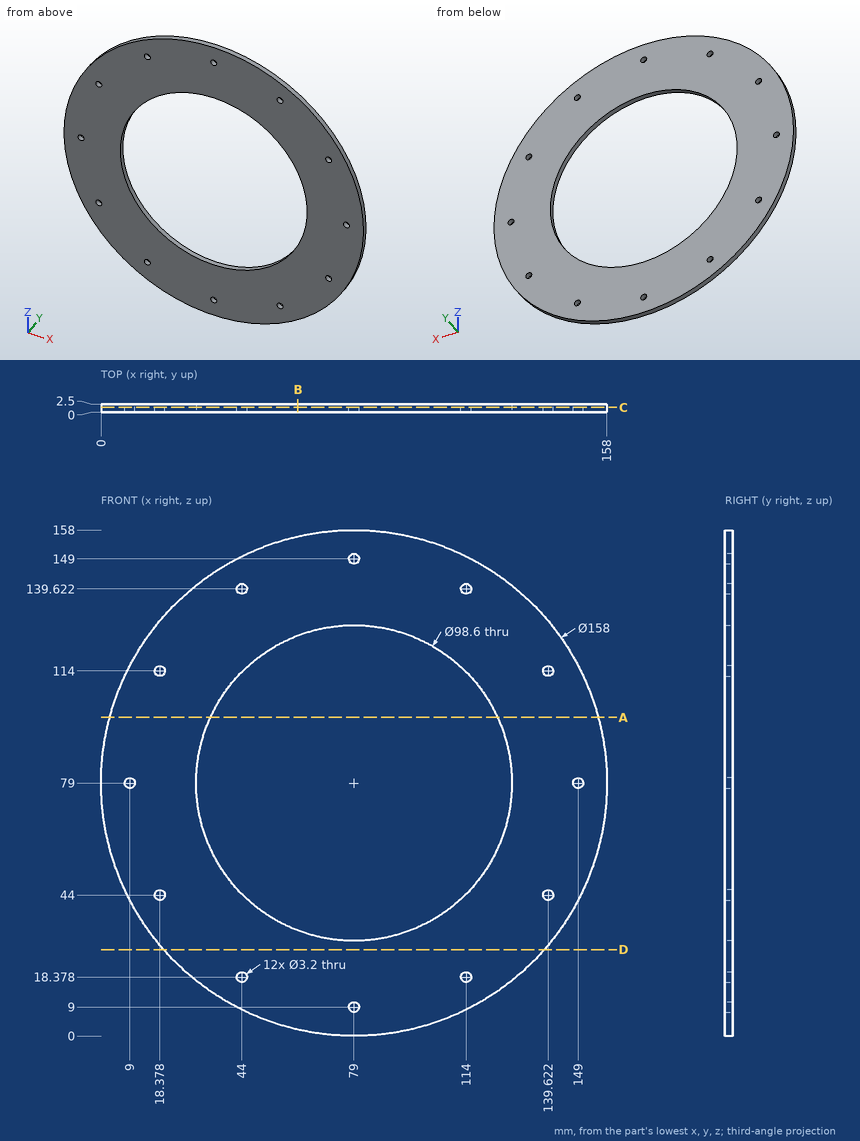
For this review, use the dimensioned drawing (mm, ordinates from the lowest corner) and the shaded views. Give positions to 0.01 mm unless a question says otherwise; leave off trailing zeros. Order: outer loops, then holes, each group sorted by start corner. A loop starts at its lowest first (then second) coordinate and runs counter-clockwise, first axis right, second up.
1) Take a section at D-D (z = 27). Give the boundary of the cut face in (x, y).
2) Insertion check: pin 1 (3.5 mm diameter, centred on x = 139.62, z = 114, fed in from -Y); pin 2 (1.9 mm diameter, centred on x = 149, z = 79, fed in from +Y); pin 3 (1 mm diameter, centred on x = 124, y = 1.5, fed in from -Z) (1 decimal); pin 4 (1.5 mm diameter, centred on y = 2, z = 52.5, fed in from -X). Each pin has a flat end and moves straight along its axis. Give the tip position at first contact, or say it passes through.
3) Wall thickness on line 1 (X direction, y = 0.5, z = 9); line 2 (X direction, y = 0.6, z = 18) (1 decimal); line 3 (X direction, y = 1.8, z = 80): over which ranges is each line inside the solid? List them lowest first.
4) Take a section at A-A (z = 99.5). Give the boundary of the cut face in (x, y), then the cut area to 3 significant figures.
5) Take a section at B-B (x = 61.5). Give the boundary of the cut face in (y, z), then the cut area to 3 significant figures.
6) Take a section at C-C (y = 1.45). State how many separate pieces and enclosed holes the cut face has, then the cut area to 3 significant figures.
Derived:
1. outline: (19.53, 0) - (138.47, 0) - (138.47, 2.5) - (19.53, 2.5) - close
2. pin 1: stops at y = 0
2. pin 2: passes through
2. pin 3: stops at z = 13.7
2. pin 4: stops at x = 4.31
3. line 1: x = 42.38 to 77.4, 80.6 to 115.62
3. line 2: x = 28.8 to 42.4, 45.6 to 112.4, 115.6 to 129.2
3. line 3: x = 0.01 to 7.75, 10.25 to 29.71, 128.29 to 147.75, 150.25 to 157.99
4. outline: (2.71, 0) - (34.16, 0) - (34.16, 2.5) - (2.71, 2.5) - close; (123.84, 0) - (155.29, 0) - (155.29, 2.5) - (123.84, 2.5) - close
4. area: 157 mm2
5. outline: (0, 1.96) - (2.5, 1.96) - (2.5, 32.91) - (0, 32.91) - close; (0, 125.09) - (2.5, 125.09) - (2.5, 156.04) - (0, 156.04) - close
5. area: 155 mm2
6. separate pieces: 1
6. enclosed holes: 13
6. area: 11,900 mm2
